from build123d import *

# Parameters (mm, degrees)
F0_W     = 48
F0_H     = 38
F1_DEPTH = 3
F2_W     = 3
F2_H     = 30
F3_DEPTH = 25


with BuildPart() as f1:
    # F0 (on Front) → F1 (new body)
    with BuildSketch(Plane.XZ):
        Polygon((-37.5, 78.245069), (-112, 78.245069), (-112, -1.754931), (-109, -1.754931), (-109, 1.745069), (-106, 1.745069), (-106, -1.754931), (61, -1.754931), (61, 1.745069), (64, 1.745069), (64, -1.754931), (67, -1.754931), (67, 78.245069), (-7.5, 78.245069), (-7.5, 81.245069), (-37.5, 81.245069), align=None)
        with Locations((-75.5, 52.745069)):
            Rectangle(F0_W, F0_H, mode=Mode.SUBTRACT)
    extrude(amount=F1_DEPTH)

    # F2 (on face) → F3 (cut)
    with BuildSketch(Plane(origin=(0, 0, 0), x_dir=(-1, 0, 0), z_dir=(0, 1, 0))):
        with Locations((-65.5, 38.245069)):
            Rectangle(F2_W, F2_H)
        with Locations((110.5, 38.245069)):
            Rectangle(F2_W, F2_H)
    extrude(amount=-F3_DEPTH, mode=Mode.SUBTRACT)


solid = f1.part
Verification items for the finished model (mm, model axes). A direction names the side the tool comes from. Give positions to 0.01 mm unless a question says otherwise; leave off trailing zeros. Loops run counter-clockwise (first coordinate to the right, second up) from the corner with the lowest first, then second, coordinate; pieces in that order, holes last.
1. Cross-section at A-A on x = -73.5. Record the cut outline in (y, z).
Derived:
outline: (-3, -1.75) - (0, -1.75) - (0, 33.75) - (-3, 33.75) - close; (-3, 71.75) - (0, 71.75) - (0, 78.25) - (-3, 78.25) - close
2. Tool access check on faces 5 (the flat face through (64, -1, 0)), 6 (the flat face through (-74, -1, 78.245)), 7 (the flat face through (66, -1, 53.245)), 8 (the flat face through (-110, -1, 53.245)), 9 (the flat face through (-76, -1, 33.745)). Record the directions out of +Z, -Z, +X, -X, +Y, -Y that give a thin tool (end or side, any length) a straight path to the whole face; none if there is none.
Derived:
face 5: -Z, +Y, -Y
face 6: +Z, -X, +Y, -Y
face 7: +X, +Y, -Y
face 8: -X, +Y, -Y
face 9: +Y, -Y
3. Cross-section at B-B on y = -1.2. Record the cut outline in (x, z).
Derived:
outline: (-112, -1.75) - (-109, -1.75) - (-109, 1.75) - (-106, 1.75) - (-106, -1.75) - (61, -1.75) - (61, 1.75) - (64, 1.75) - (64, -1.75) - (67, -1.75) - (67, 23.25) - (64, 23.25) - (64, 53.25) - (67, 53.25) - (67, 78.25) - (-7.5, 78.25) - (-7.5, 81.25) - (-37.5, 81.25) - (-37.5, 78.25) - (-112, 78.25) - (-112, 53.25) - (-109, 53.25) - (-109, 23.25) - (-112, 23.25) - close; hole (-99.5, 33.75) - (-51.5, 33.75) - (-51.5, 71.75) - (-99.5, 71.75) - close
4. Release check for a two-part mould opening along Z. For faces 1 (the flat face through (-112, -1, 11)), 2 (the flat face through (-108, -1, 1.745)), 3 (the flat face through (-110, -1, 23.245)), 4 (the flat face through (-22, -1, 81.245)) record: +Z half, -Z half, draft (parallel to the pull), parting line (faces both ways), or undercut.
Derived:
face 1: draft
face 2: -Z half
face 3: undercut
face 4: +Z half
5. Cross-section at D-D on x = 48.5. Record the cut outline in (y, z).
Derived:
outline: (-3, -1.75) - (0, -1.75) - (0, 78.25) - (-3, 78.25) - close
6. Cross-section at C-C on z = 30.5. Record the cut outline in (x, y).
Derived:
outline: (-109, -3) - (64, -3) - (64, 0) - (-109, 0) - close
7. Material ranges on probe 1 along X at (y, z) = (-0.1, 66); probe 2 along Z at (x, y) = (-95.5, -0.5); probe 3 along X at (y, z) = (-1.85, 48), recorded low to high.
Derived:
probe 1: x = -112 to -99.5, -51.5 to 67
probe 2: z = -1.75 to 33.75, 71.75 to 78.25
probe 3: x = -109 to -99.5, -51.5 to 64
8. Go/stop test with flat-tipped pins: P1, Ø1.5, axis at x = -75.5, y = -1.5, coming from the +Z side; P2, Ø0.9, axis at y = -1, z = 80, coming from the -X side. Record where each tip stops, or that it passes through.
Derived:
P1: stops at z = 78.25
P2: stops at x = -37.5
